The listing builds one solid part. Answer for the finished solid, in the listing's coordinates (mm). Face numbers are marked on the shaded views. A direction names the side the tool comes from. Round coordinates to 2 decimals unless told otherwise and drop trailing zeros. Loops run counter-clockwise (first coordinate to the right, second up) from the corner with the lowest first, then second, coordinate; pieces in that order, holes last. Notation, with made-up numbers: M -21,54 L 36,54 A12 cw 36,58 Z; hole C 82,-4 d3. An arc over 180 degrees is marked long. Answer as a JSON object with one key per item and string values.
```python
from build123d import *

# Parameters (mm, degrees)
AUFSATZ_LINEAR_AUSTRAGEN1_DEPTH      = 20
AUFSATZ_LINEAR_AUSTRAGEN1_DEPTH_BACK = 20
SCHNITT_LINEAR_AUSTRAGEN1_DEPTH      = 15
SCHNITT_LINEAR_AUSTRAGEN1_DEPTH_BACK = 15
SCHNITT_LINEAR_AUSTRAGEN2_REACH      = 62
SKIZZE3_R                            = 4
SCHNITT_LINEAR_AUSTRAGEN3_REACH      = 62
SKIZZE4_R                            = 4


with BuildPart() as part:
    # Skizze1 → Aufsatz-Linear austragen1 (new, two sides: drawn at the far end of the back side and taken through both)
    with BuildSketch(Plane(origin=(0, 0, 0), x_dir=(0, 0, -1), z_dir=(1, 0, 0)).offset(-AUFSATZ_LINEAR_AUSTRAGEN1_DEPTH_BACK)):
        Polygon((0, 0), (0, 40), (40, 0), align=None)
    extrude(amount=AUFSATZ_LINEAR_AUSTRAGEN1_DEPTH + AUFSATZ_LINEAR_AUSTRAGEN1_DEPTH_BACK)

    # Skizze2 → Schnitt-Linear austragen1 (cut, two sides: drawn at the far end of the back side and taken through both)
    with BuildSketch(Plane(origin=(0, 0, 0), x_dir=(0, 0, -1), z_dir=(1, 0, 0)).offset(-SCHNITT_LINEAR_AUSTRAGEN1_DEPTH_BACK)):
        Polygon((5, 35), (5, 5), (35, 5), align=None)
    extrude(amount=SCHNITT_LINEAR_AUSTRAGEN1_DEPTH + SCHNITT_LINEAR_AUSTRAGEN1_DEPTH_BACK, mode=Mode.SUBTRACT)

    # Skizze3 → Schnitt-Linear austragen2 (cut, up to next)
    with BuildSketch(Plane.XY, mode=Mode.PRIVATE) as schnitt_linear_austragen2_sk1:
        with Locations((0, 20)):
            Circle(SKIZZE3_R)
    schnitt_linear_austragen2_tool1 = extrude(schnitt_linear_austragen2_sk1.sketch, amount=-SCHNITT_LINEAR_AUSTRAGEN2_REACH, mode=Mode.PRIVATE) & part.part
    add(schnitt_linear_austragen2_tool1.solids().sort_by_distance((0, 20, 0))[0], mode=Mode.SUBTRACT)

    # Skizze4 → Schnitt-Linear austragen3 (cut, up to next)
    with BuildSketch(Plane.XZ, mode=Mode.PRIVATE) as schnitt_linear_austragen3_sk1:
        with Locations(Location((0, -20, 0), (0, 0, 270))):
            Circle(SKIZZE4_R)
    schnitt_linear_austragen3_tool1 = extrude(schnitt_linear_austragen3_sk1.sketch, amount=-SCHNITT_LINEAR_AUSTRAGEN3_REACH, mode=Mode.PRIVATE) & part.part
    add(schnitt_linear_austragen3_tool1.solids().sort_by_distance((0, 0, -20))[0], mode=Mode.SUBTRACT)


solid = part.part
```
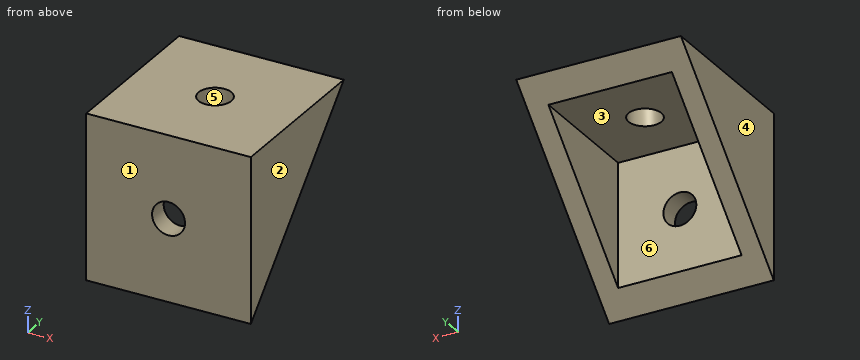
Item 1: Which of the six approach directions +Z, -Z, +X, -X, +Y, -Y give full straight-line access (tool end or side, diameter ignored) to the marked faces 5 and 6?
Values follow:
{"face 5": "+Z, -Z", "face 6": "-Z, +Y"}
Item 2: The part is cut by section C-C (y = 20). Give the vertices of the cut face in (x, z), then the cut area to 3 significant figures.
Values follow:
{"outline": "M -20,-20 L -15,-20 L -15,-5 L -4,-5 L -4,0 L -20,0 Z; M 4,-5 L 15,-5 L 15,-20 L 20,-20 L 20,0 L 4,0 Z", "area": "310 mm^2"}
Item 3: Determine the mould class of the marked faces 1, 2, 3 and 4 for opening direction X: released by +X, released by -X, zero draft, split by the parting line, or undercut.
Values follow:
{"face 1": "zero draft", "face 2": "released by +X", "face 3": "undercut", "face 4": "released by -X"}
Item 4: The part is cut by section A-A (x = 0). Give the vertices of the cut face in (y, z), then the cut area to 3 significant figures.
Values follow:
{"outline": "M 0,-40 L 5,-35 L 5,-24 L 0,-24 Z; M 0,-16 L 5,-16 L 5,-5 L 16,-5 L 16,0 L 0,0 Z; M 24,-5 L 35,-5 L 40,0 L 24,0 Z", "area": "270 mm^2"}
Item 5: Straight lines are drawn through the part: line 1 (X direction, y = 13, z = -22); line 2 (Z direction, x = 9.5, y = 8.5); line 3 (Y direction, x = 0, z = -2.65). For each, find the intervals that lie inside material, in ascending order.
Values follow:
{"line 1": "-20 to -15, 15 to 20", "line 2": "-5 to 0", "line 3": "0 to 16, 24 to 37.35"}
Item 6: The part is cut by section B-B (z = -20). Give the vertices of the cut face in (x, y), then the cut area to 3 significant figures.
Values follow:
{"outline": "M -20,0 L -4,0 L -4,5 L -15,5 L -15,20 L -20,20 Z; M 4,0 L 20,0 L 20,20 L 15,20 L 15,5 L 4,5 Z", "area": "310 mm^2"}
Item 7: Flat-ended cylindrical pins translate along their axes: P1, Ø3, axis at x = 0.5, z = -17, coming from the -Y side; P2, Ø1.5, axis at x = 11, y = 29, coming from the -Z side; P3, Ø15, axis at x = -6.5, z = -25, coming from the +Y side; P4, Ø7, axis at x = 0, z = -20, coming from the -Y side (3 decimals). Find the tip coordinate at first contact, or state that the pin passes through.
Values follow:
{"P1": "y = 0", "P2": "z = -5", "P3": "y = 5", "P4": "through"}
Item 8: The part is cut by section D-D (y = 28.5). Give the vertices of the cut face in (x, z), then the cut area to 3 significant figures.
Values follow:
{"outline": "M -20,-11.5 L -15,-11.5 L -15,-5 L 15,-5 L 15,-11.5 L 20,-11.5 L 20,0 L -20,0 Z", "area": "265 mm^2"}
